CAD build for the part. Positions are in the model's coordinates, mm. A direction names the side the tool comes from. Give positions to 0.01 mm unless a question says otherwise; leave off trailing zeros. Order: outer loops, then holes, each group sorted by start corner. A loop starts at its lowest first (then second) coordinate and runs counter-clockwise, first axis right, second up.
Item 1: Band-saw the part on C-C on y = 7.5. Give the cut face in (x, z), plus the area to 3 significant figures.
Item 2: Band-saw the part on B-B on y = 3.75. Give the cut face in (x, z).
Item 3: Band-saw the part on D-D on x = -10.5. Give the cut face in (y, z), plus the area to 3 significant figures.
Item 4: Wall check: L1, parallel to X at y = 14.25, z = -6; L2, parallel to Z at x = -13.5, y = 7.75; L3, parallel to X at y = 12.5, z = -31. Give the ranges that are in metal, low to high.
Item 5: Two-plate mould, pull along X, no slides. Class faces 3 (the cylindrical face through (0.459, 4.526, 6.656)), 4 (the flat face through (18.24, 7.4, -28.05)), 5 (the flat face through (-22.362, 7, -11)), 6 (the flat face through (0, 7, -5)): released by +X, released by -X, zero draft, split by the parting line, or undercut.
Item 6: Band-saw the part on A-A on z = -11. Give the cut face in (x, y), plus the area to 3 significant figures.
Item 7: Which spindle directions (+Z, -Z, +X, -X, +Y, -Y) get a long thin tool onto all of the face, cutting with end or side? Do faces 1 (the flat face through (-13.546, 7, -19)), 2 (the flat face through (22.638, 7, -11)). Say none if no direction does.
Item 8: Flat gauge pins, fed straight in: P1, Ø4.5, axis at x = 7.5, y = 10.5, coming from the +Z side; P2, Ø1, axis at y = 6.5, z = 5.5, coming from the -X side; P3, Ø4.5, axis at x = 3.5, y = 7.5, coming from the -Z side. Where does each tip first touch, or does it go through?
```python
from build123d import *

# Parameters (mm, degrees)
BOSS_EXTRUDE1_DEPTH = 15
SKETCH4_R           = 3
BOSS_EXTRUDE2_DEPTH = 13.5


with BuildPart() as part:
    # Sketch3 → Boss-Extrude1 (new body)
    with BuildSketch(Plane(origin=(0, 0, 0), x_dir=(1, 0, 0), z_dir=(0, 1, 0))):
        Polygon((-22.362385321, 0), (22.637614679, 0), (22.637614679, 22), (13.718917102, 34.275534099), (13.718917102, 5), (-13.545606537, 5), (-13.545606537, 34.135254916), (-22.362385321, 22), align=None)
    extrude(amount=BOSS_EXTRUDE1_DEPTH)

    # Sketch4 → Boss-Extrude2 (add)
    with BuildSketch(Plane.XY):
        with Locations(Location((0.068807339, 7.5, 0), (0, 0, 180))):
            Circle(SKETCH4_R)
    extrude(amount=BOSS_EXTRUDE2_DEPTH)


solid = part.part
```
The answers:
1. outline: (-22.36, -22) - (-13.55, -34.14) - (-13.55, -5) - (13.72, -5) - (13.72, -34.28) - (22.64, -22) - (22.64, 0) - (3.07, 0) - (3.07, 13.5) - (-2.93, 13.5) - (-2.93, 0) - (-22.36, 0) - close
1. area: 716 mm2
2. outline: (-22.36, -22) - (-13.55, -34.14) - (-13.55, -5) - (13.72, -5) - (13.72, -34.28) - (22.64, -22) - (22.64, 0) - (-22.36, 0) - close
3. outline: (0, -5) - (15, -5) - (15, 0) - (0, 0) - close
3. area: 75.0 mm2
4. L1: x = -22.36 to -13.55, 13.72 to 22.64
4. L2: z = -5 to 0
4. L3: x = -15.82 to -13.55, 13.72 to 16.1
5. face 3: split by the parting line
5. face 4: released by +X
5. face 5: released by -X
5. face 6: undercut
6. outline: (-22.36, 0) - (-13.55, 0) - (-13.55, 15) - (-22.36, 15) - close; (13.72, 0) - (22.64, 0) - (22.64, 15) - (13.72, 15) - close
6. area: 266 mm2
7. face 1: -Z, +Y, -Y
7. face 2: +Z, -Z, +X, +Y, -Y
8. P1: stops at z = 0
8. P2: stops at x = -2.89
8. P3: stops at z = -5
